```python
from build123d import *

# Parameters (mm, degrees)
SKETCH1_W                = 74.549
SKETCH1_H                = 74.549
SKETCH1_R                = 24.511
BOSS_EXTRUDE1_DEPTH      = 1.5875
BOSS_EXTRUDE1_DEPTH_BACK = 1.5875
SKETCH2_R                = 3.429
CUT_EXTRUDE1_DEPTH       = 4.175
MIRROR2_COPY_1_SKETCH_R  = 3.429
MIRROR2_COPY_1_DEPTH     = 4.175
SKETCH15_R               = 31.1531
SKETCH15_R_2             = 28.6131
BOSS_EXTRUDE11_DEPTH     = 1.5748
SKETCH14_W               = 49.149
SKETCH14_H               = 8.290530285
CUT_EXTRUDE6_DEPTH       = 2.5748
CUT_EXTRUDE6_DEPTH_BACK  = 4.175
FILLET2_R                = 3.175
CUT_EXTRUDE8_REACH       = 3.575
SKETCH18_W               = 74.549
SKETCH18_H               = 74.549
CUT_EXTRUDE9_DEPTH       = 0.8128
SKETCH19_W               = 3.81
SKETCH19_H               = 6.35
CUT_EXTRUDE10_DEPTH      = 3.3622
FILLET3_R                = 1.27
CIRPATTERN2_COUNT        = 11
FILLET3_OF_CIRPATTERN2_R = 1.27


with BuildPart() as part:
    # Sketch1 → Boss-Extrude1 (new body, two sides)
    with BuildSketch(Plane.XY) as boss_extrude1_sk:
        Rectangle(SKETCH1_W, SKETCH1_H)
        Circle(SKETCH1_R, mode=Mode.SUBTRACT)
    extrude(amount=BOSS_EXTRUDE1_DEPTH)
    extrude(boss_extrude1_sk.sketch, amount=-BOSS_EXTRUDE1_DEPTH_BACK)

    # Sketch2 → Cut-Extrude1 (cut, through all)
    with BuildSketch(Plane.XY.offset(1.5875)):
        with Locations((-31.75, 31.75)):
            Circle(SKETCH2_R)
    cut_extrude1 = extrude(amount=-CUT_EXTRUDE1_DEPTH, mode=Mode.SUBTRACT)

    # Mirror1: Cut-Extrude1 across plane
    add(cut_extrude1.mirror(Plane(origin=(0, 0, 0), x_dir=(0, 0, 1), z_dir=(1, 0, 0))), mode=Mode.SUBTRACT)

    # Mirror2: Cut-Extrude1 across plane
    add(cut_extrude1.mirror(Plane.ZX), mode=Mode.SUBTRACT)

    # Mirror2 copy 1 sketch → Mirror2 copy 1 (cut, through all)
    with BuildSketch(Plane(origin=(0, 0, 1.5875), x_dir=(-1, 0, 0), z_dir=(0, 0, 1))):
        with Locations((-31.75, 31.75)):
            Circle(MIRROR2_COPY_1_SKETCH_R)
    extrude(amount=-MIRROR2_COPY_1_DEPTH, mode=Mode.SUBTRACT)

    # Sketch15 → Boss-Extrude11 (add)
    with BuildSketch(Plane.XY.offset(1.5875)):
        Circle(SKETCH15_R)
        Circle(SKETCH15_R_2, mode=Mode.SUBTRACT)
    extrude(amount=BOSS_EXTRUDE11_DEPTH)

    # Sketch14 → Cut-Extrude6 (cut, two sides)
    with BuildSketch(Plane.XY.offset(1.5875)) as cut_extrude6_sk:
        with Locations((0, 35.069765143)):
            Rectangle(SKETCH14_W, SKETCH14_H)
    extrude(amount=CUT_EXTRUDE6_DEPTH, mode=Mode.SUBTRACT)
    extrude(cut_extrude6_sk.sketch, amount=-CUT_EXTRUDE6_DEPTH_BACK, mode=Mode.SUBTRACT)

    # Fillet2
    fillet2_edges = [part.edges().sort_by_distance(p)[0] for p in [
        (-24.5745, 30.9245, 0),
        (24.5745, 30.9245, 0),
    ]]
    fillet(fillet2_edges, radius=FILLET2_R)

    # Sketch17 → Cut-Extrude8 (cut, up to next)
    with BuildSketch(Plane.XY.offset(1.5875), mode=Mode.PRIVATE) as cut_extrude8_sk1:
        with BuildLine():
            Line((-1.5875, 24.754637718), (-1.5875, 33.858616052))
            ThreePointArc((-1.5875, 33.858616052), (0, 35.446116052), (1.5875, 33.858616052))
            Line((1.5875, 33.858616052), (1.5875, 24.754637718))
            ThreePointArc((1.5875, 24.754637718), (0, 23.167137718), (-1.5875, 24.754637718))
        make_face()
    cut_extrude8_tool1 = extrude(cut_extrude8_sk1.sketch, amount=CUT_EXTRUDE8_REACH, mode=Mode.PRIVATE) & part.part
    add(cut_extrude8_tool1.solids().sort_by_distance((0, 29.306627, 1.5875))[0], mode=Mode.SUBTRACT)

    # Sketch18 → Cut-Extrude9 (cut)
    with BuildSketch(Plane(origin=(0, 0, -1.5875), x_dir=(-1, 0, 0), z_dir=(0, 0, -1))):
        Rectangle(SKETCH18_W, SKETCH18_H)
    extrude(amount=-CUT_EXTRUDE9_DEPTH, mode=Mode.SUBTRACT)

    # Sketch19 → Cut-Extrude10 (cut, through all)
    with BuildSketch(Plane.XY.offset(1.5875)):
        with Locations((0, -23.495)):
            Rectangle(SKETCH19_W, SKETCH19_H)
    cut_extrude10 = extrude(amount=-CUT_EXTRUDE10_DEPTH, mode=Mode.SUBTRACT)

    # Fillet3
    fillet3_edges = [part.edges().sort_by_distance(p)[0] for p in [
        (-1.905, -26.67, 0.4064),
        (1.905, -26.67, 0.4064),
    ]]
    fillet(fillet3_edges, radius=FILLET3_R)

    # CirPattern2: Cut-Extrude10 ×11 about axis
    cirpattern2_axis = Axis((0, 0, 0), (0, 0, 1))
    for i in range(1, CIRPATTERN2_COUNT):
        add(cut_extrude10.rotate(cirpattern2_axis, i * 360 / CIRPATTERN2_COUNT), mode=Mode.SUBTRACT)

    # Fillet3 of CirPattern2
    fillet3_of_cirpattern2_edges = [part.edges().sort_by_distance(p)[0] for p in [
        (12.816302621, -23.466152478, 0.4064),
        (16.021478582, -21.406310963, 0.4064),
        (23.468519716, -12.811967348, 0.4064),
        (25.051250916, -9.346269446, 0.4064),
        (26.669647622, 1.90992689, 0.4064),
        (26.127428088, 5.681146584, 0.4064),
        (21.403350846, 16.025432835, 0.4064),
        (18.90833145, 18.904838713, 0.4064),
        (9.341641406, 25.052977086, 0.4064),
        (5.685973176, 26.126378127, 0.4064),
        (-5.685973176, 26.126378127, 0.4064),
        (-9.341641406, 25.052977086, 0.4064),
        (-18.90833145, 18.904838713, 0.4064),
        (-21.403350846, 16.025432835, 0.4064),
        (-26.127428088, 5.681146584, 0.4064),
        (-26.669647622, 1.90992689, 0.4064),
        (-25.051250916, -9.346269446, 0.4064),
        (-23.468519716, -12.811967348, 0.4064),
        (-16.021478582, -21.406310963, 0.4064),
        (-12.816302621, -23.466152478, 0.4064),
    ]]
    fillet(fillet3_of_cirpattern2_edges, radius=FILLET3_OF_CIRPATTERN2_R)


solid = part.part
```
The listing builds one solid part. Answer for the finished solid, in the listing's coordinates (mm). A direction names the side the tool comes from. Round coordinates to 2 decimals unless told otherwise and drop trailing zeros. Order: outer loops, then holes, each group sorted by start corner. A loop starts at its lowest first (then second) coordinate and runs counter-clockwise, first axis right, second up. Notation, with made-up numbers: (39.25, 48) -> (48.25, 48) arc R34 cw to (48.25, 85) -> close; hole circle Ø9 at (83.5, 73.25). An arc over 180 degrees is marked (long way). Answer as CSV lines item,"result". Start each with the question number.
(1) A tool of negligible diameter and unlimited length cuts with its end or side. For faces 4 (the face through (12.942, -22.955, 0.39)), 5 (the face through (9, -23, 1.588)), 6 (the face through (-24.574, 36, 0)), from which of +Z, -Z, +X, -X, +Y, -Y can it reach the whole face along a straight path? Write none if from no direction.
(2) Find the intervals of material crossed by probe 1 along Y at (x, z) = (31.75, 0.5); probe 2 along Y at (x, z) = (-0.5, -0.05); probe 3 along Y at (x, z) = (0, 2.85), in increasing order. Write a range as from..to.
(3) For a pull along X with two mould halves and no side action, classify faces 1 (the face through (-31, 37.274, 0)), 2 (the face through (24.553, -9.517, 0.39)), 3 (the face through (-37.274, -1, 0)) as +X half, -X half, draft (parallel to the pull), parting line (faces both ways), or undercut.
(4) A flat-ended cylindrical pin translates along its axis: pin 1 Ø0.6 at (x, z) = (0, 0) entering from +Y. Find the tip coordinate at first contact, or state that the pin passes through.
(5) The part is cut by section B-B (z = 0.2). Count the separate pieces of the cut face and the enclosed holes in it, then the cut area to 3 significant figures.
(6) The part is cut by section A-A (y = -16). Determine the outline of the cut face in (x, z), then the cut area to 3 significant figures.
Evaluation:
1,face 4,"+Z, -Z"
1,face 5,"+Z"
1,face 6,"+Z, -Z, +Y"
2,probe 1,"-37.27..-35.18, -28.32..28.32, 35.18..37.27"
2,probe 2,"-37.27..-26.67, 24.51..30.92"
2,probe 3,"-31.15..-28.61"
3,face 1,"draft"
3,face 2,"undercut"
3,face 3,"-X half"
4,pin 1,"y = 30.92"
5,separate pieces,"1"
5,enclosed holes,"5"
5,area,"3,130 mm²"
6,outline,"(-37.27, -0.77) -> (-18.57, -0.77) -> (-18.57, 1.59) -> (-23.72, 1.59) -> (-23.72, 3.16) -> (-26.73, 3.16) -> (-26.73, 1.59) -> (-37.27, 1.59) -> close; (18.57, -0.77) -> (37.27, -0.77) -> (37.27, 1.59) -> (26.73, 1.59) -> (26.73, 3.16) -> (23.72, 3.16) -> (23.72, 1.59) -> (18.57, 1.59) -> close"
6,area,"97.9 mm²"
